Part model, mm, in its own coordinate system. Face numbers are marked on the shaded views. A direction names the side the tool comes from. Coordinates: 2 decimals unless noted, no trailing zeros. Loops run counter-clockwise (first coordinate to the right, second up) from the corner with the lowest first, then second, coordinate; pieces in that order, holes last. Notation, with made-up numbers: (13.5, 59.5) -> (61.5, 59.5) arc R21 cw to (61.5, 92.5) -> close; hole circle Ø3 at (-13, 62). An arc over 180 degrees is marked (long way). Use one line per item in the form item = value. Start each with the question number.
(1) Band-saw the part on B-B on y = -17.5. Give the cut face in (x, z) (3 decimals), then the cut area to 3 significant figures.
(2) Band-saw the part on D-D on z = 4.75. Count the separate pieces of the cut face and the enclosed holes in it, then the cut area to 3 significant figures.
(3) Band-saw the part on A-A on x = -12. Give the cut face in (y, z) (3 decimals).
(4) Drill centre lines: L1, parallel to X at y = 4, z = 4.75; L2, parallel to Y at x = -30, z = 4.25; L3, parallel to Y at x = 17, z = 4.75. Where is each one in solid material? Low to high. Write a range as [from, to].
(5) Band-saw the part on C-C on x = 2.5. Give the cut face in (y, z) (3 decimals), then the cut area to 3 significant figures.
(6) Pin check, flat tip, straight feed: P1, Ø3, axis at x = 20, y = 6.25, coming from the +Z side. Stop position of the tip, or through.
(7) Mould opens along Y. For the marked faces 1, 2 and 3 say: +Y half, -Y half, draft (parallel to the pull), parting line (faces both ways), or undercut.
(8) 3-axis set-ups, long thin cutter, end or side, ignore diameter. For the marked faces 4 and 5: which of +Z, -Z, +X, -X, +Y, -Y reach the whole face in a straight line?
```python
from build123d import *

# Parameters (mm, degrees)
F0_W     = 70
F0_H     = 76
F0_R     = 2.25
F0_R_2   = 1.375
F0_R_3   = 0.875
F0_R_4   = 5.625
F0_R_5   = 6.5
F1_DEPTH = 13
F2_R     = 1.375
F2_R_2   = 0.875
F2_R_3   = 5.625
F2_W     = 50
F2_H     = 8.5
F3_DEPTH = 10
F4_R     = 3


with BuildPart() as f1:
    # F0 (on Top) → F1 (new body)
    with BuildSketch(Plane.XY):
        Rectangle(F0_W, F0_H)
        with Locations((-30, -32)):
            Circle(F0_R, mode=Mode.SUBTRACT)
        with Locations((30, -32)):
            Circle(F0_R, mode=Mode.SUBTRACT)
        with Locations((2.5, -17.5)):
            Circle(F0_R_2, mode=Mode.SUBTRACT)
        with Locations((18.5, -9)):
            Circle(F0_R_3, mode=Mode.SUBTRACT)
        with Locations((-12, 2)):
            Circle(F0_R_4, mode=Mode.SUBTRACT)
        with Locations((-30, 32)):
            Circle(F0_R, mode=Mode.SUBTRACT)
        with Locations((-8.0413195181, 32.907142101)):
            Circle(F0_R_2, mode=Mode.SUBTRACT)
        with Locations((8.0413195181, 15.092857899)):
            Circle(F0_R_2, mode=Mode.SUBTRACT)
        with Locations((20, 6.25)):
            Circle(F0_R_3, mode=Mode.SUBTRACT)
        with Locations((0, 24)):
            Circle(F0_R_5, mode=Mode.SUBTRACT)
        with Locations((14.25, 20.5)):
            Circle(F0_R_3, mode=Mode.SUBTRACT)
        with Locations((30, 32)):
            Circle(F0_R, mode=Mode.SUBTRACT)
    extrude(amount=F1_DEPTH)

    # F2 (on face) → F3 (cut)
    with BuildSketch(Plane.XY.offset(13)):
        with BuildLine():
            Line((-25, 27), (-32.5, 27))
            Line((-32.5, 27), (-32.5, -27))
            Line((-32.5, -27), (-25, -27))
            Line((-25, -27), (25, -27))
            Line((25, -27), (32.5, -27))
            Line((32.5, -27), (32.5, 27))
            Line((32.5, 27), (25, 27))
            Line((25, 27), (5.7662812973, 27))
            ThreePointArc((5.7662812973, 27), (6.3139064149, 25.5442104078), (6.5, 24))
            ThreePointArc((6.5, 24), (-1.5442104078, 17.6860935851), (-5.7662812973, 27))
            Line((-5.7662812973, 27), (-25, 27))
        make_face()
        with Locations((2.5, -17.5)):
            Circle(F2_R, mode=Mode.SUBTRACT)
        with Locations((18.5, -9)):
            Circle(F2_R_2, mode=Mode.SUBTRACT)
        with Locations((-12, 2)):
            Circle(F2_R_3, mode=Mode.SUBTRACT)
        with Locations((8.0413195181, 15.092857899)):
            Circle(F2_R, mode=Mode.SUBTRACT)
        with Locations((20, 6.25)):
            Circle(F2_R_2, mode=Mode.SUBTRACT)
        with Locations((14.25, 20.5)):
            Circle(F2_R_2, mode=Mode.SUBTRACT)
        with BuildLine():
            Line((-25, 35.5), (-25, 27))
            Line((-25, 27), (-5.7662812973, 27))
            ThreePointArc((-5.7662812973, 27), (0, 30.5), (5.7662812973, 27))
            Line((5.7662812973, 27), (25, 27))
            Line((25, 27), (25, 35.5))
            Line((25, 35.5), (-25, 35.5))
        make_face()
        with Locations((-8.0413195181, 32.907142101)):
            Circle(F2_R, mode=Mode.SUBTRACT)
        with Locations((0, -31.25)):
            Rectangle(F2_W, F2_H)
    extrude(amount=-F3_DEPTH, mode=Mode.SUBTRACT)

    # F4
    f4_edges = [f1.edges().sort_by_distance(p)[0] for p in [
        (-25, 27, 8),
        (25, 27, 8),
        (-25, -27, 8),
        (25, -27, 8),
        (32.5, -27, 8),
        (32.5, 27, 8),
        (25, 35.5, 8),
        (-25, 35.5, 8),
        (-32.5, 27, 8),
        (-32.5, -27, 8),
        (-25, -35.5, 8),
        (25, -35.5, 8),
    ]]
    fillet(f4_edges, radius=F4_R)


solid = f1.part
```
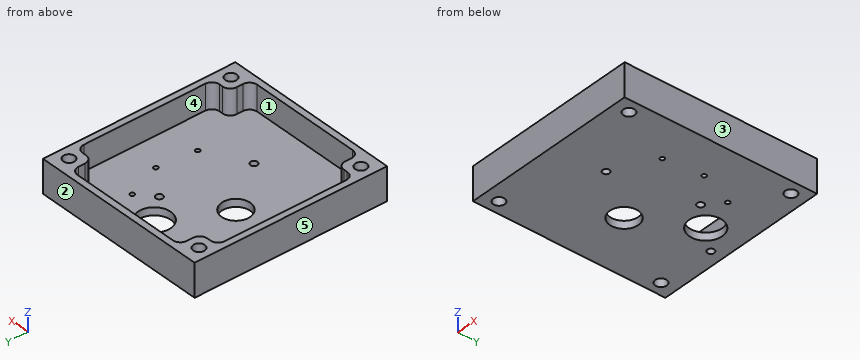
A:
q1.outline = (-35, 0) -> (1.125, 0) -> (1.125, 3) -> (-32.5, 3) -> (-32.5, 13) -> (-35, 13) -> close; (3.875, 0) -> (35, 0) -> (35, 13) -> (32.5, 13) -> (32.5, 3) -> (3.875, 3) -> close
q1.area = 252 mm²
q2.separate_pieces = 1
q2.enclosed_holes = 5
q2.area = 904 mm²
q3.outline = (-38, 0) -> (-3.625, 0) -> (-3.625, 3) -> (-35.5, 3) -> (-35.5, 13) -> (-38, 13) -> close; (7.625, 0) -> (38, 0) -> (38, 13) -> (35.5, 13) -> (35.5, 3) -> (7.625, 3) -> close
q4.L1 = [-35, -32.5], [32.5, 35]
q4.L2 = [-38, -34.25], [-29.75, -26.96], [26.96, 29.75], [34.25, 38]
q4.L3 = [-38, -35.5], [35.5, 38]
q5.outline = (-38, 0) -> (-18.875, 0) -> (-18.875, 3) -> (-35.5, 3) -> (-35.5, 13) -> (-38, 13) -> close; (-16.125, 0) -> (18, 0) -> (18, 3) -> (-16.125, 3) -> close; (30, 0) -> (38, 0) -> (38, 13) -> (35.5, 13) -> (35.5, 3) -> (30, 3) -> close
q5.area = 234 mm²
q6.P1 = 3
q7.face_1 = undercut
q7.face_2 = +Y half
q7.face_3 = draft
q8.face_4 = +Z
q8.face_5 = +Z, -Z, -X, +Y, -Y
